Geometry: final body of the model. Coordinates: model frame, mm. Face numbers are marked on the shaded views. A direction names the side the tool comes from. Give positions to 0.01 mm unless a question says otherwise; leave off trailing zeros. Loops run counter-clockwise (first coordinate to the right, second up) from the corner with the lowest first, then second, coordinate; pieces in that order, holes last.
from build123d import *

# Parameters (mm, degrees)
F2_DEPTH = 1.6
F3_DEPTH = 5.1
F4_DEPTH = 17.2
F1_R     = 2.05
F1_W     = 2.5
F1_H     = 7.1
F1_W_2   = 7.1
F1_H_2   = 2.5
F6_DEPTH = 8.4
F1_W_3   = 6.4
F1_H_3   = 4.6
F7_DEPTH = 9.2
F8_DEPTH = 18.8
F1_W_4   = 3.1
F1_H_4   = 1.3
F1_W_5   = 4.6
F1_H_5   = 2.4
F1_W_6   = 16.6
F1_H_6   = 2.6
F9_DEPTH = 1.5


# Not quite as in the source:
# - a fillet or chamfer that OpenCascade refuses, or shapes differently, is made with other operations: its cross-section is extruded or revolved along the edge and cut away or added


with BuildPart() as f2:
    # F0 (on Front) → F2 (new body)
    with BuildSketch(Plane.XZ):
        Polygon((16.3, -12.05), (16.3, 12.05), (12.05, 12.05), (12.05, 0), (12.05, -12.05), align=None)
        with BuildLine():
            Line((12.05, 0), (12.05, 12.05))
            Line((12.05, 12.05), (0, 12.05))
            ThreePointArc((0, 12.05), (8.5206367133, 8.5206367133), (12.05, 0))
        make_face()
        with BuildLine():
            ThreePointArc((-12.05, 0), (-8.5206367133, 8.5206367133), (0, 12.05))
            Line((0, 12.05), (-12.05, 12.05))
            Line((-12.05, 12.05), (-12.05, 0))
        make_face()
        with BuildLine():
            ThreePointArc((12.05, 0), (8.5206367133, 8.5206367133), (0, 12.05))
            ThreePointArc((0, 12.05), (-8.5206367133, 8.5206367133), (-12.05, 0))
            ThreePointArc((-12.05, 0), (-8.5206367125, -8.5206367141), (2.1e-09, -12.05))
            ThreePointArc((2.1e-09, -12.05), (8.5206367141, -8.5206367125), (12.05, 0))
        make_face()
        with BuildLine():
            Line((12.05, -12.05), (12.05, 0))
            ThreePointArc((12.05, 0), (8.5206367141, -8.5206367125), (2.1e-09, -12.05))
            Line((2.1e-09, -12.05), (12.05, -12.05))
        make_face()
        Polygon((-12.05, 0), (-12.05, 12.05), (-16.3, 12.05), (-16.3, -12.05), (-12.05, -12.05), align=None)
        with BuildLine():
            ThreePointArc((2.1e-09, -12.05), (-8.5206367125, -8.5206367141), (-12.05, 0))
            Line((-12.05, 0), (-12.05, -12.05))
            Line((-12.05, -12.05), (2.1e-09, -12.05))
        make_face()
    extrude(amount=-F2_DEPTH)

    # F0 (on Front) → F3 (join)
    with BuildSketch(Plane.XZ):
        with BuildLine():
            ThreePointArc((2.1e-09, -12.05), (-8.5206367125, -8.5206367141), (-12.05, 0))
            Line((-12.05, 0), (-12.05, -12.05))
            Line((-12.05, -12.05), (2.1e-09, -12.05))
        make_face()
        with BuildLine():
            ThreePointArc((-12.05, 0), (-8.5206367133, 8.5206367133), (0, 12.05))
            Line((0, 12.05), (-12.05, 12.05))
            Line((-12.05, 12.05), (-12.05, 0))
        make_face()
        with BuildLine():
            ThreePointArc((12.05, 0), (8.5206367133, 8.5206367133), (0, 12.05))
            ThreePointArc((0, 12.05), (-8.5206367133, 8.5206367133), (-12.05, 0))
            ThreePointArc((-12.05, 0), (-8.5206367125, -8.5206367141), (2.1e-09, -12.05))
            ThreePointArc((2.1e-09, -12.05), (8.5206367141, -8.5206367125), (12.05, 0))
        make_face()
        with BuildLine():
            Line((12.05, 0), (12.05, 12.05))
            Line((12.05, 12.05), (0, 12.05))
            ThreePointArc((0, 12.05), (8.5206367133, 8.5206367133), (12.05, 0))
        make_face()
        with BuildLine():
            Line((12.05, -12.05), (12.05, 0))
            ThreePointArc((12.05, 0), (8.5206367141, -8.5206367125), (2.1e-09, -12.05))
            Line((2.1e-09, -12.05), (12.05, -12.05))
        make_face()
    extrude(amount=-F3_DEPTH)

    # F0 (on Front) → F4 (join)
    with BuildSketch(Plane.XZ):
        with BuildLine():
            ThreePointArc((12.05, 0), (8.5206367133, 8.5206367133), (0, 12.05))
            ThreePointArc((0, 12.05), (-8.5206367133, 8.5206367133), (-12.05, 0))
            ThreePointArc((-12.05, 0), (-8.5206367125, -8.5206367141), (2.1e-09, -12.05))
            ThreePointArc((2.1e-09, -12.05), (8.5206367141, -8.5206367125), (12.05, 0))
        make_face()
    extrude(amount=-F4_DEPTH)

    # F5: fillet of radius 12 on 1 edges, made by hand

    # F5_s1 → F5_t2 (revolve, cut)
    with BuildSketch(Plane.YZ):
        with BuildLine():
            ThreePointArc((5.2, -12.05), (13.6852813742, -8.5352813742), (17.2, -0.05))
            Line((17.2, -0.05), (17.2, -12.05))
            Line((17.2, -12.05), (5.2, -12.05))
        make_face()
    revolve(axis=Axis((0, 17.2, 0), (0, -1, 0)), mode=Mode.SUBTRACT)

    # F1 (on Front) → F6 (join)
    with BuildSketch(Plane.XZ):
        with Locations((-14.25, 10)):
            Circle(F1_R)
        with Locations((14.25, 10)):
            Circle(F1_R)
        with Locations((14.25, -10)):
            Circle(F1_R)
        with Locations((-8.15, -10)):
            Circle(F1_R)
        with Locations((-15.05, -7.7)):
            Rectangle(F1_W, F1_H)
        with Locations((-0.05, 10.8)):
            Rectangle(F1_W_2, F1_H_2)
    extrude(amount=F6_DEPTH)

    # F1 (on Front) → F7 (join)
    with BuildSketch(Plane.XZ):
        with Locations((-1.4, -8.75)):
            Rectangle(F1_W_3, F1_H_3)
        with Locations((6.7, -8.75)):
            Rectangle(F1_W_3, F1_H_3)
    extrude(amount=F7_DEPTH)

    # F1 (on Front) → F8 (join)
    with BuildSketch(Plane.XZ):
        with Locations((-0.05, 10.8)):
            Rectangle(F1_W_2, F1_H_2)
    extrude(amount=F8_DEPTH)

    # F1 (on Front) → F9 (join)
    with BuildSketch(Plane.XZ):
        with Locations((-14.75, -2.4)):
            Rectangle(F1_W_4, F1_H_4)
        with Locations((12, 3.65)):
            Rectangle(F1_W_5, F1_H_5)
        with Locations((8, -3.8)):
            Rectangle(F1_W_6, F1_H_4)
        with Locations((-14.75, 5.45)):
            Rectangle(F1_W_4, F1_H_6)
    extrude(amount=F9_DEPTH)


solid = f2.part
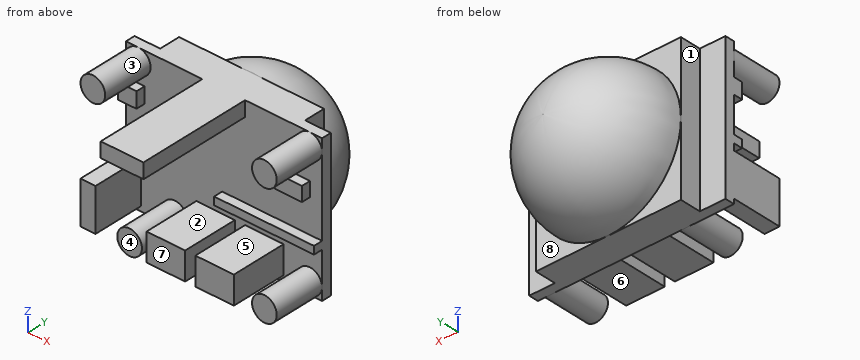
Item 1: Section query A-A on y = -14.5. Return loops of the section in (x, z), plus the area to 4 significant figures.
Values follow:
outline: (-3.6, 9.55) - (3.5, 9.55) - (3.5, 12.05) - (-3.6, 12.05) - close
area: 17.75 mm2
Item 2: Ray query, probe 1 along X at (y, z) = (-7.5, -10.75); probe 2 along Z at (x, y) = (-3, -2.5); probe 3 along X at (y, z) = (3.5, -1). Return the intervals inside material, ascending.
Values follow:
probe 1: x = -16.3 to -13.8, -10.06 to -6.24, -4.6 to 1.8, 3.5 to 9.9, 12.34 to 16.16
probe 2: z = -11.05 to -6.45, 9.55 to 12.05
probe 3: x = -12.05 to 12.05
Item 3: Pin query (flat end, axial travel): pin 1 (6 mm diameter, centred on x = -5.5, z = -5, fed in from +Y); pin 2 (1.5 mm diameter, centred on x = 2, z = 1, fed in from +Y); pin 3 (8 mm diameter, centred on x = 3.5, z = -1, fed in from -Y). Return the tip coordinate at first contact, or that it passes through.
Values follow:
pin 1: stops at y = 16.37
pin 2: stops at y = 17.11
pin 3: stops at y = -1.5
Item 4: Draft query along X for the marked faces 1, 2 and 3. Return one class per face: +X half, -X half, draft (parallel to the pull), parting line (faces both ways), or undercut.
Values follow:
face 1: -X half
face 2: draft
face 3: undercut
Item 5: Set-up query: the marked faces 4, 5, 6, 7 and 8. Return all of +Z, -Z, +X, -X, +Y, -Y with unobstructed straight access to the full face (end or side cutting, diameter ignored); none if empty.
Values follow:
face 4: +Z, -Z, -X, -Y
face 5: +X, -Y
face 6: -Z, -Y
face 7: -Z, +X, -X, -Y
face 8: -Z, +X, +Y
